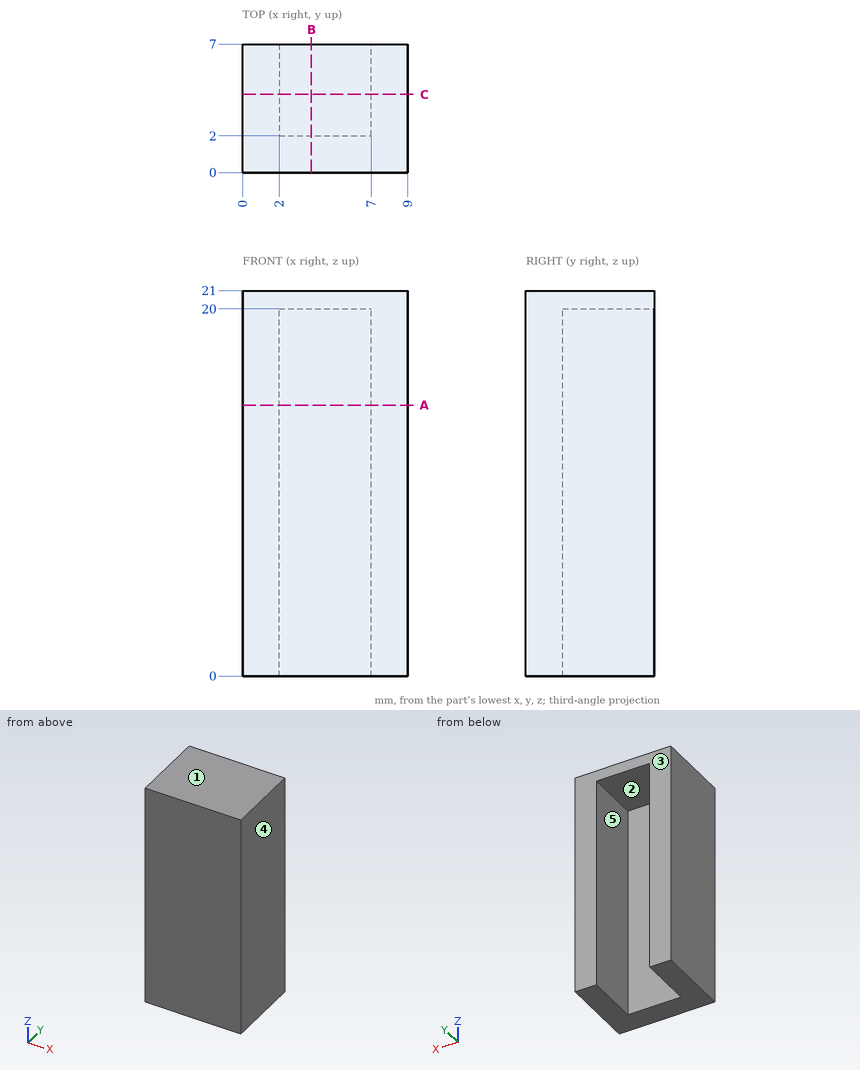
Input: dimensioned drawing with shaded views. Units: mm. Origin: part minimum x, y, z. A direction names the side the tool comes from. Round coordinates to 2 decimals unless told otherwise and drop trailing zeros. Order: outer loops, then holes, each group sorted by start corner. A loop starts at its lowest first (then second) coordinate and runs counter-clockwise, first axis right, second up. Notation, with made-up numbers: (16.25, -4) - (42.25, -4) arc R22 ccw to (42.25, 25) - close; hole circle Ø6 at (-13.5, 51). An arc over 180 degrees is marked (long way). Write item = value, one per line. Start each with the question number.
Q1. Cut plane B-B on x = 3.75. Return the cut outline in (y, z).
Q2. Access query for the marked faces 1 and 2. Directions: +Z, -Z, +X, -X, +Y, -Y. A direction counts if a zero-diameter tool reaches every point of the face in a straight line with its end or side. Return the directions, or none.
Q3. Pin query (flat end, axial travel): pin 1 (2 mm diameter, centred on y = 4, z = 4.5, fed in from -X); pin 2 (1.5 mm diameter, centred on x = 4.5, z = 13.5, fed in from +Y). Return the tip coordinate at first contact, or that it passes through.
Q4. Cut plane C-C on y = 4.25. Return the cut outline in (x, z).
Q5. Cut plane A-A on z = 14.75. Return the cut outline in (x, y), and give its area (3 significant figures).
Q6. Ray query, line 1 (X direction, y = 3.5, z = 14.75); line 2 (Y direction, x = 4, z = 3); line 3 (Z direction, x = 4, y = 5.25). Return the intervals inside material, ascending. Write a range as from..to.
Q7. Pull-direction query (X, two-part tool) for the marked faces 3, 4 and 5; classes: +X half, -X half, draft (parallel to the pull), parting line (faces both ways), or undercut.
Outcome:
q1.outline = (0, 0) - (2, 0) - (2, 20) - (7, 20) - (7, 21) - (0, 21) - close
q2.face_1 = +Z, +X, -X, +Y, -Y
q2.face_2 = -Z, +Y
q3.pin_1 = 0
q3.pin_2 = 2
q4.outline = (0, 0) - (2, 0) - (2, 20) - (7, 20) - (7, 0) - (9, 0) - (9, 21) - (0, 21) - close
q5.outline = (0, 0) - (9, 0) - (9, 7) - (7, 7) - (7, 2) - (2, 2) - (2, 7) - (0, 7) - close
q5.area = 38.0 mm^2
q6.line_1 = 0..2, 7..9
q6.line_2 = 0..2
q6.line_3 = 20..21
q7.face_3 = draft
q7.face_4 = +X half
q7.face_5 = undercut
